from build123d import *

# Parameters (mm, degrees)
SKETCH_1_W          = 11
SKETCH_1_H          = 14
SKETCH_1_R          = 2.1
EXTRUDE_1_DEPTH     = 8
CUT_EXTRUDE_1_DEPTH = 18


with BuildPart() as part:
    # Эскиз1 → Вытянуть1 (new body)
    with BuildSketch(Plane.XY):
        with Locations((5.5, 7)):
            Rectangle(SKETCH_1_W, SKETCH_1_H)
        with Locations((5.5, 7)):
            Circle(SKETCH_1_R, mode=Mode.SUBTRACT)
    extrude(amount=EXTRUDE_1_DEPTH)

    # Эскиз2 → Вырез-Вытянуть1 (cut)
    with BuildSketch(Plane(origin=(11, 0, 0), x_dir=(0, 0, -1), z_dir=(1, 0, 0))):
        with BuildLine():
            Line((-5.5, 15.242713302), (-2.5, 15.242713302))
            Line((-2.5, 15.242713302), (-2.5, 10.75))
            ThreePointArc((-2.5, 10.75), (-4.00000012, 9.25), (-5.5, 10.750000239))
            Line((-5.5, 10.750000239), (-5.5, 15.242713302))
        make_face()
        with BuildLine():
            Line((-5.5, -1.965553789), (-2.5, -1.965553789))
            Line((-2.5, -1.965553789), (-2.5, 3.25))
            ThreePointArc((-2.5, 3.25), (-3.999999879, 4.75), (-5.5, 3.250000241))
            Line((-5.5, 3.250000241), (-5.5, -1.965553789))
        make_face()
    extrude(amount=-CUT_EXTRUDE_1_DEPTH, mode=Mode.SUBTRACT)


solid = part.part
Work out the finished part from the listing and answer in its coordinate system (mm). A direction names the side the tool comes from. Give positions to 0.01 mm unless a question says otherwise; leave off trailing zeros. Loops run counter-clockwise (first coordinate to the right, second up) from the corner with the lowest first, then second, coordinate; pieces in that order, holes last. Notation, with made-up numbers: (3.25, 24) -> (14.25, 24) arc R13 cw to (14.25, 42) -> close; hole circle Ø4 at (53, 59.5). An arc over 180 degrees is marked (long way). Use a Markdown table: item, result. Add a question column.
1. Find the intervals of material crossed by probe 1 along Z at (x, y) = (4.25, 13.25); probe 2 along Y at (x, z) = (5.5, 5.75); probe 3 along Y at (x, z) = (5.5, 5.25), in increasing order.
2. Determine the mould class of faces 1 (the cylindrical face through (5.58, 9.25, 3.97)), 2 (the flat face through (0, 7, 4)), 3 (the flat face through (4, 9, 0)) for opening direction Z: released by +Z, released by -Z, zero draft, split by the parting line, or undercut.
3. For faces 4 (the flat face through (6, 2, 5.5)), 5 (the flat face through (6, 12, 2.5)), 6 (the flat face through (5, 14, 7)), determine the directions among +Z, -Z, +X, -X, +Y, -Y from which every point of the face is accessible in a straight line to the end or side of a thin tool.
4. Section A-A on y = 2.5 is taken. Determine the outline of the cut face in (x, z).
5. Section D-D on x = 1.5 is taken. Determine the outline of the cut face in (y, z), and give its area (3 significant figures).
6. Section C-C on x = 7 is taken. Determine the outline of the cut face in (y, z).
7. Flat-ended cylindrical pins translate along their axes: pin 1 Ø2.5 at (x, y) = (6, 1.5) entering from -Z; pin 2 Ø3.5 at (x, y) = (5.5, 7) entering from +Z. Find the tip coordinate at first contact, or state that the pin passes through.
8. Section B-B on z = 1.25 is taken. Determine the outline of the cut face in (x, y), and give its area (3 significant figures).
Results below:
| question | item | result |
|---|---|---|
| 1 | probe 1 | z = 0 to 2.5, 5.5 to 8 |
| 1 | probe 2 | y = 0 to 4.9, 9.1 to 14 |
| 1 | probe 3 | y = 4.08 to 4.9, 9.1 to 9.92 |
| 2 | face 1 | undercut |
| 2 | face 2 | zero draft |
| 2 | face 3 | released by -Z |
| 3 | face 4 | +X, -X, -Y |
| 3 | face 5 | +X, -X, +Y |
| 3 | face 6 | +Z, -Z, +X, -X, +Y |
| 4 | outline | (0, 0) -> (11, 0) -> (11, 2.5) -> (0, 2.5) -> close; (0, 5.5) -> (11, 5.5) -> (11, 8) -> (0, 8) -> close |
| 5 | outline | (0, 0) -> (14, 0) -> (14, 2.5) -> (10.75, 2.5) arc R1.5 cw to (10.75, 5.5) -> (14, 5.5) -> (14, 8) -> (0, 8) -> (0, 5.5) -> (3.25, 5.5) arc R1.5 cw to (3.25, 2.5) -> (0, 2.5) -> close |
| 5 | area | 85.4 mm^2 |
| 6 | outline | (0, 0) -> (5.53, 0) -> (5.53, 8) -> (0, 8) -> (0, 5.5) -> (3.25, 5.5) arc R1.5 cw to (3.25, 2.5) -> (0, 2.5) -> close; (8.47, 0) -> (14, 0) -> (14, 2.5) -> (10.75, 2.5) arc R1.5 cw to (10.75, 5.5) -> (14, 5.5) -> (14, 8) -> (8.47, 8) -> close |
| 7 | pin 1 | stops at z = 0 |
| 7 | pin 2 | passes through |
| 8 | outline | (0, 0) -> (11, 0) -> (11, 14) -> (0, 14) -> close; hole circle Ø4.2 at (5.5, 7) |
| 8 | area | 140 mm^2 |
